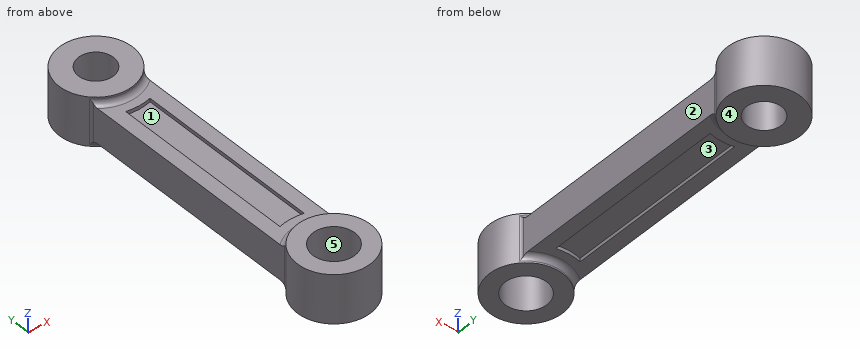
Autodesk Inventor part; units mm, degrees
ref_plane "YZ Plane" through (0, 0, 0) normal (1, 0, 0) x (0, 1, 0)
ref_plane "XZ Plane" through (0, 0, 0) normal (0, 1, 0) x (-1, 0, 0)
ref_plane "XY Plane" through (0, 0, 0) normal (0, 0, 1) x (1, 0, 0)
sketch "Sketch1" plane through (0, 0, 0) normal (0, 0, 1) x (1, 0, 0)
  line L0 (0, 0) -> (0, 40) construction
  circle A0 centre (0, 40) radius 2.5
  circle A1 centre (0, 40) radius 5.25
  circle A2 centre (0, 0) radius 3
  circle A3 centre (0, 0) radius 5.25
  dimension "d0" = 40
  dimension "d1" = 5
  dimension "d2" = 10.5
  dimension "d3" = 6
  dimension "d4" = 10.5
extrude "Extrusion1" add sketch "Sketch1" along normal mid plane 7
sketch "Sketch2" plane through (0, 0, 0) normal (0, 0, 1) x (1, 0, 0)
  circle A0 centre (0, 40) radius 2.5
  circle A1 centre (0, 40) radius 5.25
  circle A2 centre (0, 0) radius 3
  circle A3 centre (0, 0) radius 5.25
  circle A4 centre (0, 0) radius 3
  line L0 (0, 40) -> (0, 0) construction
  line L1 (-3.75, 36.3258) -> (-3.75, 3.6742)
  line L2 (3.75, 36.3258) -> (3.75, 3.6742)
  point P0 (-3.75, 40)
  point P1 (-3.75, 0)
  point P2 (3.75, 40)
  point P3 (3.75, 0)
  dimension "d7" = 3.75
extrude "Extrusion2" add sketch "Sketch2" along normal mid plane 5 contours A1 L2 A3 L1
sketch "Sketch3" plane through (0, 0, 2.5) normal (0, 0, 1) x (1, 0, 0)
  line L0 (-3.75, 36.3258) -> (-3.75, 3.6742)
  line L1 (-3.75, 36.3258) -> (-3.75, 3.6742)
  arc A0 (3.75, 3.6742) -> (-3.75, 3.6742) centre (0, 0) ccw
  line L2 (3.75, 3.6742) -> (3.75, 36.3258)
  arc A1 (-3.75, 36.3258) -> (3.75, 36.3258) centre (0, 40) ccw
  line L3 (1.75, 32.9644) -> (1.75, 7.0356)
  arc A2 (1.75, 7.0356) -> (-1.75, 7.0356) centre (0, 0) ccw
  line L4 (-1.75, 7.0356) -> (-1.75, 32.9644)
  arc A3 (-1.75, 32.9644) -> (1.75, 32.9644) centre (0, 40) ccw
  dimension "d10" = 2
extrude "Extrusion3" cut sketch "Sketch3" against normal blind 0.5 contours L3 A2 L4 A3
mirror "Mirror1" about plane through (0, 0, 0) normal (0, 0, 1) of "Extrusion3"
fillet "Fillet1" radius 0.75 8 edges at (0, 34.75, 2.5) (3.75, 36.3258, 0) (0, 34.75, -2.5) (-3.75, 36.3258, 0) (3.75, 3.6742, 0) (0, 5.25, -2.5) (-3.75, 3.6742, 0) (0, 5.25, 2.5)
properties part number "Component 6 (Connecting Rod)"
Could you check a few things on this model? Use its own coordinates, in mm. Face numbers are marked on the shaded views. A direction names the side the tool comes from. Round coordinates to 2 decimals unless told otherwise and drop trailing zeros. Loops run counter-clockwise (first coordinate to the right, second up) from the corner with the lowest first, then second, coordinate; pieces in that order, holes last. Notation, with made-up numbers: (87, -11) -> (118, -11) arc R29 ccw to (118, 22) -> close; hole circle Ø11 at (33, 15.25). An arc over 180 degrees is marked (long way). Use CSV: the item, a comma, the result in double quotes.
(1) Suppose I cut it at B-B on x = 0. Give the number of separate pieces and of enclosed holes in the cut face, plus the area to 3 significant figures.
Return value:
separate pieces,"3"
enclosed holes,"0"
area,"192 mm²"
(2) Suppose I cut it at A-A on y = 40. Write out the boundary of the cut face in (x, z), plus the area to 3 significant figures.
Return value:
outline,"(-5.25, -3.5) -> (-2.5, -3.5) -> (-2.5, 3.5) -> (-5.25, 3.5) -> close; (2.5, -3.5) -> (5.25, -3.5) -> (5.25, 3.5) -> (2.5, 3.5) -> close"
area,"38.5 mm²"
(3) Suppose I cut it at D-D on x = 4.75. Write out the boundary of the cut face in (y, z), plus the area to 3 significant figures.
Return value:
outline,"(-2.24, -3.5) -> (2.24, -3.5) -> (2.24, 3.5) -> (-2.24, 3.5) -> close; (37.76, -3.5) -> (42.24, -3.5) -> (42.24, 3.5) -> (37.76, 3.5) -> close"
area,"62.6 mm²"
(4) If I drill on probe 1 along Y at (x, z) = (0, 0.5); probe 2 along Y at (x, z) = (-1.75, -3); probe 3 along X at (y, z) = (23.5, -0.5), over which ranges is the centre line in solid material (lowest first)? Write a range as [from, to].
Return value:
probe 1,"y = [-5.25, -3], [3, 37.5], [42.5, 45.25]"
probe 2,"y = [-4.95, -2.44], [2.44, 5], [35, 38.21], [41.79, 44.95]"
probe 3,"x = [-3.75, 3.75]"
(5) For the marked faces 1, 2 and 3, which set-ups out of +Z, -Z, +X, -X, +Y, -Y let a thin tool reach every point of the face, with its end or its side?
Return value:
face 1,"+Z"
face 2,"+Z, -Z, +X"
face 3,"-Z"
(6) If we mould it in two halves opening along Y, with no side actions, what happens to the marked faces 4 and 5? For each: +Y half, -Y half, draft (parallel to the pull), parting line (faces both ways), or undercut.
Return value:
face 4,"draft"
face 5,"undercut"
(7) Will these pins go through, and if not, where does the flat tip stop? pin 1 Ø1.8 at (x, y) = (-0.5, 19) entering from -Z; pin 2 Ø2.5 at (y, z) = (26, 0.5) entering from +X; pin 3 Ø1.8 at (x, y) = (0, 23) entering from +Z.
Return value:
pin 1,"stops at z = -2"
pin 2,"stops at x = 3.75"
pin 3,"stops at z = 2"
(8) Suppose I cut it at C-C on z = -1.25. Write out the boundary of the cut face in (x, y), plus the area to 3 significant figures.
Return value:
outline,"(-3.94, 3.47) arc R5.25 ccw (long way) to (3.94, 3.47) arc R0.75 cw to (3.75, 3.97) -> (3.75, 36.03) arc R0.75 cw to (3.94, 36.53) arc R5.25 ccw (long way) to (-3.94, 36.53) arc R0.75 cw to (-3.75, 36.03) -> (-3.75, 3.97) arc R0.75 cw to start; hole circle Ø6 at (0, 0); hole circle Ø5 at (0, 40)"
area,"354 mm²"
